Here's how the part is built. I have some questions about the finished solid (model axes, mm). A direction names the side the tool comes from. Coordinates: 2 decimals unless noted, no trailing zeros. Write each loop counter-clockwise with the first axis right and the second up, starting at its lowest first coordinate (ties: lowest second). Pieces come first, ordered by that corner, then holes. Notation, with made-up numbers: (88.5, 13) - (113.5, 13) arc R17 ccw to (113.5, 28) - close; hole circle Ø10 at (23, -37). An arc over 180 degrees is marked (long way). Answer in a Markdown table with one row per item. Add a question column.
Item 1: Which directions (+Z, -Z, +X, -X, +Y, -Y) give clear straight access to the entire face, cutting with the end or side of a thin tool? Please do faces 4 (the face through (8, 8, 2.54)), 5 (the face through (8, 7, 12.7)).
Item 2: Imagine slicing it at D-D (z = 1). Please give me the cut outline in (x, y) (3 decimals).
Item 3: I'm going to push flat-ended pins straight in: pin 1 (5 mm diameter, centred on y = 20.32, z = 6.35, fed in from +X); pin 2 (12 mm diameter, centred on x = 9, y = 11, fed in from +Z). Where does each tip first touch, or does it pass through?
Item 4: We'd pull the mould along Y, two halves only. Please class faces 1 (the face through (9.132, 9.283, 1.252)), 2 (the face through (1.9, 18.8, 5.2)), 3 (the face through (7, 7, 10.16)): +Y half, -Y half, draft (parallel to the pull), parting line (faces both ways), or undercut.
Item 5: Imagine slicing it at A-A (x = 20.32). Please give me the cut outline in (y, z) (3 decimals).
Item 6: Imagine slicing it at B-B (z = 6.35). Please give me the cut outline in (x, y) (3 decimals), plus the area to 3 significant figures.
Item 7: If I drill on probe 1 along Z at (x, y) = (1, 20.32) (3 decimals); probe 2 along Y at (x, z) = (11.25, 10), over which ranges is the centre line in solid material (lowest first)? Write a range as from..to.
from build123d import *

# Parameters (mm, degrees)
F1_DEPTH  = 12.7
F4_DEPTH  = 2.54
F6_R      = 1.905
F7_DEPTH  = 25.4
F8_DEPTH  = 2.54
F9_R      = 1.905
F10_DEPTH = 25.4


with BuildPart() as f1:
    # F0 (on Top) → F1 (new body)
    with BuildSketch(Plane.XY):
        Polygon((0, 25.4), (0, 0), (25.4, 0), (25.4, 3.81), (3.81, 3.81), (3.81, 25.4), align=None)
    extrude(amount=F1_DEPTH)

    # F2 (on face) → F4 (join)
    with BuildSketch(Plane.XY.offset(12.7)):
        Polygon((14.605, 3.81), (3.81, 14.605), (3.81, 3.81), align=None)
    extrude(amount=-F4_DEPTH)

    # F6 (on face) → F7 (cut)
    with BuildSketch(Plane.YZ.offset(3.81)):
        with Locations((20.32, 6.35)):
            Circle(F6_R)
    extrude(amount=-F7_DEPTH, mode=Mode.SUBTRACT)

    # F5 (on face) → F8 (join)
    with BuildSketch(Plane(origin=(0, 0, 0), x_dir=(1, 0, 0), z_dir=(0, 0, -1))):
        Polygon((3.81, -14.605), (14.605, -3.81), (3.81, -3.81), align=None)
    extrude(amount=-F8_DEPTH)

    # F9 (on face) → F10 (cut)
    with BuildSketch(Plane(origin=(0, 3.81, 0), x_dir=(-1, 0, 0), z_dir=(0, 1, 0))):
        with Locations((-20.32, 6.35)):
            Circle(F9_R)
    extrude(amount=-F10_DEPTH, mode=Mode.SUBTRACT)


solid = f1.part
Here are the results:
| question | item | result |
|---|---|---|
| 1 | face 4 | +X, +Y |
| 1 | face 5 | +Z, +X, -X, +Y, -Y |
| 2 | outline | (0, 0) - (25.4, 0) - (25.4, 3.81) - (14.605, 3.81) - (3.81, 14.605) - (3.81, 25.4) - (0, 25.4) - close |
| 3 | pin 1 | stops at x = 3.81 |
| 3 | pin 2 | stops at z = 12.7 |
| 4 | face 1 | +Y half |
| 4 | face 2 | undercut |
| 4 | face 3 | draft |
| 5 | outline | (0, 0) - (3.81, 0) - (3.81, 4.445) - (0, 4.445) - close; (0, 8.255) - (3.81, 8.255) - (3.81, 12.7) - (0, 12.7) - close |
| 6 | outline | (0, 0) - (18.415, 0) - (18.415, 3.81) - (3.81, 3.81) - (3.81, 18.415) - (0, 18.415) - close; (0, 22.225) - (3.81, 22.225) - (3.81, 25.4) - (0, 25.4) - close; (22.225, 0) - (25.4, 0) - (25.4, 3.81) - (22.225, 3.81) - close |
| 6 | area | 150 mm2 |
| 7 | probe 1 | z = 0..4.445, 8.255..12.7 |
| 7 | probe 2 | y = 0..3.81 |
